Part model, mm, in its own coordinate system. Round coordinates to 2 decimals unless told otherwise and drop trailing zeros. Loops run counter-clockwise (first coordinate to the right, second up) from the corner with the lowest first, then second, coordinate; pieces in that order, holes last.
from build123d import *

# Parameters (mm, degrees)
SKETCH1_R          = 48.5
SKETCH1_R_2        = 27.5
BASE_EXTRUDE_DEPTH = 7


with BuildPart() as part:
    # Sketch1 → Base-Extrude (new body)
    with BuildSketch(Plane.XY):
        with BuildLine():
            Line((-6.343577624, -161.833816921), (-7.052214122, -148.618592863))
            ThreePointArc((-7.052214122, -148.618592863), (20.539062499, -101.208107275), (75.015436064, -107.639080177))
            Line((75.015436064, -107.639080177), (115.358185855, -141.490666647))
            ThreePointArc((115.358185855, -141.490666647), (133.059494125, -142.650871687), (139.488887394, -126.117714323))
            Line((139.488887394, -126.117714323), (119.384026274, -51.085351142))
            ThreePointArc((119.384026274, -51.085351142), (117.893575292, -46.990370726), (115.714681724, -43.216416361))
            Line((115.714681724, -43.216416361), (57.3406431, 40.150350545))
            ThreePointArc((57.3406431, 40.150350545), (-22.829860749, 66.172482636), (-69.899577583, -3.748206743))
            Line((-69.899577583, -3.748206743), (-54.913923642, -283.212748636))
            ThreePointArc((-54.913923642, -283.212748636), (-36.27490207, -323.547473625), (5, -340))
            Line((5, -340), (46.927843862, -340))
            ThreePointArc((46.927843862, -340), (64.292661629, -338.480775301), (81.129858195, -333.969262079))
            Line((81.129858195, -333.969262079), (106.154745303, -324.860948055))
            ThreePointArc((106.154745303, -324.860948055), (123.808625639, -311.314649231), (130.5, -290.092321086))
            Line((130.5, -290.092321086), (130.5, -269.907678914))
            ThreePointArc((130.5, -269.907678914), (123.808625639, -248.685350769), (106.154745303, -235.139051945))
            Line((106.154745303, -235.139051945), (26.483684912, -206.14115743))
            ThreePointArc((26.483684912, -206.14115743), (3.409872911, -188.922008159), (-6.343577624, -161.833816921))
        make_face()
        Circle(SKETCH1_R, mode=Mode.SUBTRACT)
        with Locations((5, -280)):
            Circle(SKETCH1_R_2, mode=Mode.SUBTRACT)
    extrude(amount=BASE_EXTRUDE_DEPTH)


solid = part.part
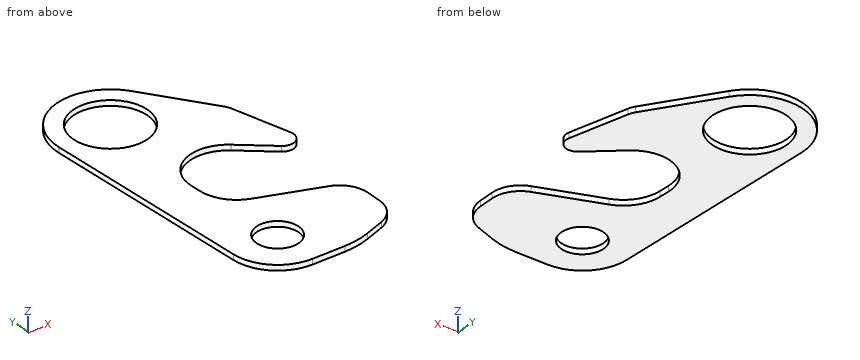
1) Drop flat-ended pins along their axis: pin 1 Ø1.5 at (x, y) = (98, -281) entering from -Z; pin 2 Ø2 at (x, z) = (51.5, 6) entering from +Y; pin 3 Ø4 at (x, z) = (81.5, 5) entering from -Y; pin 4 Ø1.5 at (y, z) = (-49.5, 5) entering from +X. Give the stop position or say it passes through.
Values:
pin 1: stops at z = 0
pin 2: stops at y = 48.47
pin 3: stops at y = -334.55
pin 4: stops at x = 119.14
2) Slice it at B-B, the plane y = 21. Give the cut face in (x, z).
Values:
outline: (-66.78, 0) - (-43.72, 0) - (-43.72, 7) - (-66.78, 7) - close; (43.72, 0) - (70.75, 0) - (70.75, 7) - (43.72, 7) - close
3) Slice it at A-A, the plane z = 5.5. Give the cut face in (x, y).
Values:
outline: (-69.9, -3.75) - (-54.91, -283.21) arc R60 ccw to (5, -340) - (46.93, -340) arc R100 ccw to (81.13, -333.97) - (106.15, -324.86) arc R37 ccw to (130.5, -290.09) - (130.5, -269.91) arc R37 ccw to (106.15, -235.14) - (26.48, -206.14) arc R50 cw to (-6.34, -161.83) - (-7.05, -148.62) arc R50 cw to (75.02, -107.64) - (115.36, -141.49) arc R15 ccw to (139.49, -126.12) - (119.38, -51.09) arc R25 ccw to (115.71, -43.22) - (57.34, 40.15) arc R70 ccw to start; hole circle Ø97 at (0, 0); hole circle Ø55 at (5, -280)
4) Slice it at D-D, the plane x = 86. Give the cut face in (y, z).
Values:
outline: (-332.2, 0) - (-227.8, 0) - (-227.8, 7) - (-332.2, 7) - close; (-116.86, 0) - (-0.78, 0) - (-0.78, 7) - (-116.86, 7) - close
5) Wall check: line 1 along Y through (x, z) = (-10.5, 4.25); line 2 along Y through (x, z) = (5, 4.75); line 3 along Y through (x, z) = (24.5, 6.25). Give the ranges that are in metal, low to high.
Values:
line 1: y = -337.96 to -302.72, -257.28 to -47.35, 47.35 to 69.21
line 2: y = -340 to -307.5, -252.5 to -190.96, -113.3 to -48.24, 48.24 to 69.82
line 3: y = -340 to -299.39, -260.61 to -205.37, -99.44 to -41.86, 41.86 to 65.57
6) Slice it at C-C, the plane x = 0. Give the cut face in (y, z).
Values:
outline: (-339.79, 0) - (-307.04, 0) - (-307.04, 7) - (-339.79, 7) - close; (-252.96, 0) - (-183.66, 0) - (-183.66, 7) - (-252.96, 7) - close; (-120.22, 0) - (-48.5, 0) - (-48.5, 7) - (-120.22, 7) - close; (48.5, 0) - (70, 0) - (70, 7) - (48.5, 7) - close
